Geometry check sheet. Reference: the model listing, model coordinates, mm. Coordinates: 2 decimals unless noted, no trailing zeros. Loops run counter-clockwise (first coordinate to the right, second up) from the corner with the lowest first, then second, coordinate; pieces in that order, holes last. Notation, with made-up numbers: (51.5, -2.5) -> (59.5, -2.5) arc R25 ccw to (59.5, 17.5) -> close; hole circle Ø2 at (72.25, 50). An arc over 180 degrees is marked (long way). Answer as a JSON object with one key per item and string values.
from build123d import *

# Parameters (mm, degrees)
BOSS_EXTRUDE1_DEPTH = 32.9
CUT_EXTRUDE1_DEPTH  = 275.9
BOSS_EXTRUDE2_DEPTH = 17.9


with BuildPart() as part:
    # Sketch1 → Boss-Extrude1 (new body)
    with BuildSketch(Plane(origin=(0, 0, 0), x_dir=(1, 0, 0), z_dir=(0, 1, 0))):
        Polygon((0, 244.7), (-32.901678529, 211.798321471), (-32.901678529, 32.901678529), (0, 0), align=None)
    extrude(amount=BOSS_EXTRUDE1_DEPTH)

    # Sketch2 → Cut-Extrude1 (cut)
    with BuildSketch(Plane.XY):
        Polygon((0, 32.9), (-32.901678529, 0), (-32.901678529, 32.9), align=None)
    extrude(amount=-CUT_EXTRUDE1_DEPTH, mode=Mode.SUBTRACT)

    # Sketch3 → Boss-Extrude2 (add)
    with BuildSketch(Plane.XZ):
        Polygon((0, 0), (-32.901678529, -32.901678529), (-32.901678529, -211.798321471), (0, -244.7), align=None)
    extrude(amount=BOSS_EXTRUDE2_DEPTH)


solid = part.part
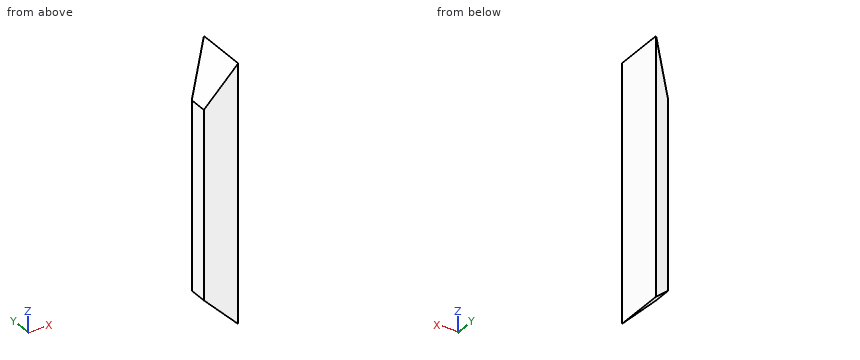
1. Depth check by flat-ended pin: P1, Ø3, axis at x = -15, z = -195, coming from the +Y side; P2, Ø8, axis at x = -11, y = -8, coming from the +Z side; P3, Ø6, axis at x = -19, y = -7.5, coming from the -Z side. Enter the tip coordinate at first touch or a pass-through.
Evaluation:
{"P1": "stops at y = 19.4", "P2": "stops at z = -7", "P3": "stops at z = -228.7"}
2. Section check B-B, the plane y = -6.5. Record the boundary of the cut face in (x, z), then the cut area to 3 significant figures.
Evaluation:
{"outline": "(-32.9, -211.8) -> (0, -244.7) -> (0, 0) -> (-32.9, -32.9) -> close", "area": "6,970 mm^2"}
3. Section check A-A, the plane z = -179. Record the boundary of the cut face in (x, y).
Evaluation:
{"outline": "(-32.9, -17.9) -> (0, -17.9) -> (0, 32.9) -> (-32.9, 0) -> close"}
4. Thickness scan on probe 1 along Y at (x, z) = (-9, -11); probe 2 along X at (y, z) = (30.5, -231); probe 3 along X at (y, z) = (-4.5, -220.5). Record the ranges inside material, lowest first. Write a range as from..to.
Evaluation:
{"probe 1": "y = -17.9..23.9", "probe 2": "x = -2.4..0", "probe 3": "x = -24.2..0"}
